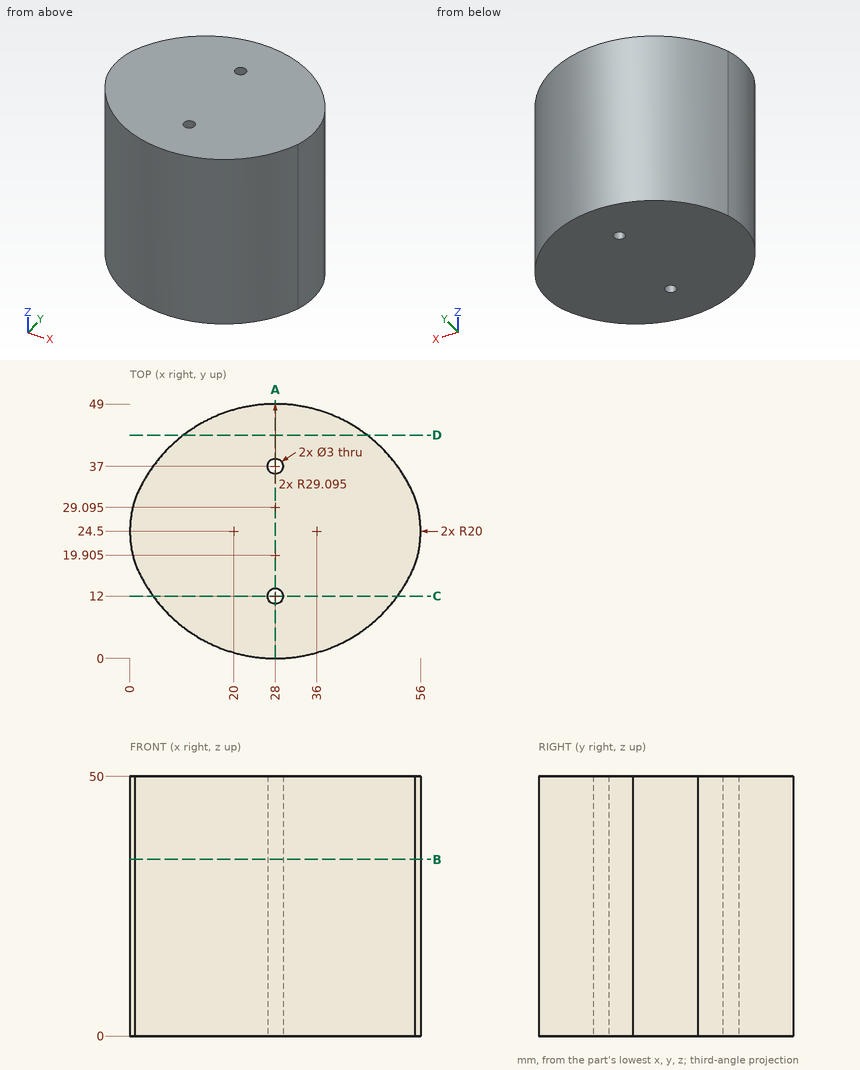
Geometry check sheet. Reference: drawing and pictorial views, mm from the part's lowest x, y, z. Coordinates: 2 decimals unless noted, no trailing zeros. Loops run counter-clockwise (first coordinate to the right, second up) from the corner with the lowest first, then second, coordinate; pieces in that order, holes last. Notation, with made-up numbers: (58, 3) -> (93, 3) arc R35 ccw to (93, 41) -> close; hole circle Ø5 at (-32, 69). An arc over 180 degrees is marked (long way). Put each result on its own line as item: value.
1) Cross-section at D-D on y = 43. Record the boundary of the cut face in (x, z).
Result set:
outline: (10.3, 0) -> (45.7, 0) -> (45.7, 50) -> (10.3, 50) -> close
2) Cross-section at A-A on x = 28. Record the boundary of the cut face in (y, z), plus the area to 3 significant figures.
Result set:
outline: (0, 0) -> (10.5, 0) -> (10.5, 50) -> (0, 50) -> close; (13.5, 0) -> (35.5, 0) -> (35.5, 50) -> (13.5, 50) -> close; (38.5, 0) -> (49, 0) -> (49, 50) -> (38.5, 50) -> close
area: 2,150 mm^2
3) Cross-section at B-B on z = 34. Count the separate pieces of the cut face and the enclosed holes in it, plus the area to 3 significant figures.
Result set:
separate pieces: 1
enclosed holes: 2
area: 2,100 mm^2
4) Gauge pin test, flat ends, axial feed: pin 1 Ø6 at (x, z) = (6.5, 18) entering from +Y; pin 2 Ø2.5 at (x, y) = (28, 37) entering from +Z; pin 3 Ø12 at (y, z) = (5.5, 13) entering from +X; pin 4 Ø6 at (y, z) = (17.5, 12) entering from +X. Record the tip position at first contact, or that the pin passes through.
Result set:
pin 1: stops at y = 42.36
pin 2: passes through
pin 3: stops at x = 51.17
pin 4: stops at x = 55.6
5) Thickness scan on line 1 (X direction, y = 12.5, z = 25) (1 decimal); line 2 (X direction, y = 16.5, z = 22); line 3 (X direction, y = 22.5, z = 32.5). Record the ranges inside material, lowest first.
Result set:
line 1: x = 4.1 to 26.6, 29.4 to 51.9
line 2: x = 1.77 to 54.23
line 3: x = 0.1 to 55.9
6) Cross-section at C-C on y = 12. Record the boundary of the cut face in (x, z), plus the area to 3 significant figures.
Result set:
outline: (4.46, 0) -> (26.5, 0) -> (26.5, 50) -> (4.46, 50) -> close; (29.5, 0) -> (51.54, 0) -> (51.54, 50) -> (29.5, 50) -> close
area: 2,200 mm^2
